Autodesk Inventor part; units mm, degrees
ref_plane "YZ Plane" through (0, 0, 0) normal (1, 0, 0) x (0, 1, 0)
ref_plane "XZ Plane" through (0, 0, 0) normal (0, 1, 0) x (-1, 0, 0)
ref_plane "XY Plane" through (0, 0, 0) normal (0, 0, 1) x (1, 0, 0)
sketch "Sketch1" plane through (0, 0, 0) normal (1, 0, 0) x (0, 1, 0)
  line L0 (0, 0) -> (4, 0)
  line L1 (4, 0) -> (6, 2)
  line L2 (6, 2) -> (6, 6)
  line L3 (6, 6) -> (4, 6)
  line L4 (4, 6) -> (4, 10)
  line L5 (4, 10) -> (0, 10)
  line L6 (0, -2) -> (0, 12)
  line L7 (0, 0) -> (-4, 0)
  line L8 (-4, 0) -> (-6, 2)
  line L9 (-6, 2) -> (-6, 6)
  line L10 (-6, 6) -> (-4, 6)
  line L11 (-4, 6) -> (-4, 10)
  line L12 (-4, 10) -> (0, 10)
  dimension "d0" = 10
  dimension "d1" = 45
  dimension "d4" = 2
  dimension "d6" = 6
  dimension "d19" = 12
  dimension "d20" = 8
extrude "Extrusion1" add sketch "Sketch1" along normal mid plane 13
sketch "Sketch2" plane through (6.5, -4, 10) normal (0, 0, 1) x (0, 1, 0)
  point P0 (4, 6.5)
hole "Hole1" at (0, 0, 10) direction (0, 0, -1) diameter 4.917 end through all
chamfer "Chamfer1" distance 0.5415 angle 45 2 edges at (0, 2.4585, 10) (0, 2.4585, 0)
properties part number "T-Nutenstein 8 - M6" material "Steel"
Can you work these out from the model? Positions are in its coordinate system, mm. A direction names the side the tool comes from. Give positions to 0.01 mm unless a question says otherwise; leave off trailing zeros. Write each loop counter-clockwise with the first axis right and the second up, starting at its lowest first coordinate (ties: lowest second). Pieces come first, ordered by that corner, then holes. Notation, with made-up numbers: (-9.75, 70.25) -> (31.25, 70.25) arc R32 cw to (31.25, 107.25) -> close; hole circle Ø4 at (89, 49.25). An arc over 180 degrees is marked (long way). Write item = value, one per line.
(1) Suppose I cut it at B-B on y = 0. Write out the boundary of the cut face in (x, z).
Worked out:
outline = (-6.5, 0) -> (-3, 0) -> (-2.46, 0.54) -> (-2.46, 9.46) -> (-3, 10) -> (-6.5, 10) -> close; (2.46, 0.54) -> (3, 0) -> (6.5, 0) -> (6.5, 10) -> (3, 10) -> (2.46, 9.46) -> close
(2) Suppose I cut it at C-C on z = 4. Write out the boundary of the cut face in (x, y).
Worked out:
outline = (-6.5, -6) -> (6.5, -6) -> (6.5, 6) -> (-6.5, 6) -> close; hole circle Ø4.92 at (0, 0)
(3) I'm going to push flat-ended pins straight in: P1, Ø4, axis at x = 0, y = 0, coming from the -Z side; P2, Ø4.5, axis at x = 0.5, z = 8.5, coming from the +Y side; P3, Ø1.6, axis at x = 0.5, y = 5, coming from the +Z side; P4, Ø1, axis at x = -3.5, z = 7.5, coming from the -Y side. Where does each tip first touch, or does it pass through?
Worked out:
P1 = through
P2 = 4
P3 = 6
P4 = -4
(4) Suppose I cut it at A-A on x = 0. Write out the boundary of the cut face in (y, z), then the cut area to 3 significant figures.
Worked out:
outline = (-6, 2) -> (-4, 0) -> (-3, 0) -> (-2.46, 0.54) -> (-2.46, 9.46) -> (-3, 10) -> (-4, 10) -> (-4, 6) -> (-6, 6) -> close; (2.46, 0.54) -> (3, 0) -> (4, 0) -> (6, 2) -> (6, 6) -> (4, 6) -> (4, 10) -> (3, 10) -> (2.46, 9.46) -> close
area = 50.2 mm^2
(5) Suppose I cut it at D-D on x = 5.5. Write out the boundary of the cut face in (y, z).
Worked out:
outline = (-6, 2) -> (-4, 0) -> (4, 0) -> (6, 2) -> (6, 6) -> (4, 6) -> (4, 10) -> (-4, 10) -> (-4, 6) -> (-6, 6) -> close
(6) For faces 1 (the face through (-3, 1, 10)), 2 (the face through (0, 5, 6)), 3 (the face through (0, -4, 8)), which set-ups out of +Z, -Z, +X, -X, +Y, -Y let a thin tool reach every point of the face, with its end or its side?
Worked out:
face_1 = +Z, +X, -X, +Y, -Y
face_2 = +Z, +X, -X, +Y
face_3 = +Z, +X, -X, -Y
(7) I need wall thicknesses on probe 1 along X at (y, z) = (0, 3.25); probe 2 along Y at (x, z) = (0, 4); probe 3 along Y at (x, z) = (-4.5, 7.25). Which ranges of each line are inside material? Lowest first, please. Write a range as from..to.
Worked out:
probe_1 = -6.5..-2.46, 2.46..6.5
probe_2 = -6..-2.46, 2.46..6
probe_3 = -4..4
(8) Thinking about a two-plate mould opening in Y: for faces 4 (the face through (-0.738, -2.345, 4.938)), 5 (the face through (0, -5, 6)), 6 (the face through (0, -5, 1)), which applies, released by +Y, released by -Y, zero draft, split by the parting line, or undercut?
Worked out:
face_4 = undercut
face_5 = zero draft
face_6 = released by -Y
